Check sheet for the drawn part. Datum: minimum x, y, z corner. Units: mm. A direction names the side the tool comes from. Coordinates: 2 decimals unless noted, no trailing zeros. Loops run counter-clockwise (first coordinate to the right, second up) from the corner with the lowest first, then second, coordinate; pieces in that order, holes last. Notation, with made-up numbers: (60, 7.25) - (89, 7.25) arc R34 ccw to (89, 43.25) - close; hole circle Ø8 at (-4.5, 22.5). An arc over 180 degrees is marked (long way). Answer as CSV lines item,"result". Start each with the question number.
1. Cross-section at B-B (x = 9). Enter the section's corners in (y, z).
2. Cross-section at D-D (z = 4.25). Enter the section's corners in (x, y), plus the area to 3 significant figures.
3. Cross-section at A-A (y = 8). Enter the section's corners in (x, z), plus the area to 3 significant figures.
4. Cross-section at C-C (z = 6.25). Enter the section's corners in (x, y).
5. Gauge pin test, flat ends, axial feed: P1, Ø4, axis at x = 19, z = 5, coming from the -Y side; P2, Ø5, axis at x = 19.5, y = 17.5, coming from the +Z side. Record the tip position at first contact, or that the pin passes through.
6. Material ranges on line 1 (Y direction, x = 5, z = 0.4); line 2 (Y direction, x = 26.5, z = 4.5); line 3 (Z direction, x = 25, y = 24.5), recorded low to high. Write a range as [from, to].
7. Set-up check for the marked faces 1 and 2: record each of +Z, -Z, +X, -X, +Y, -Y from which the full face is reachable in a straight line by a thin tool's end or side.
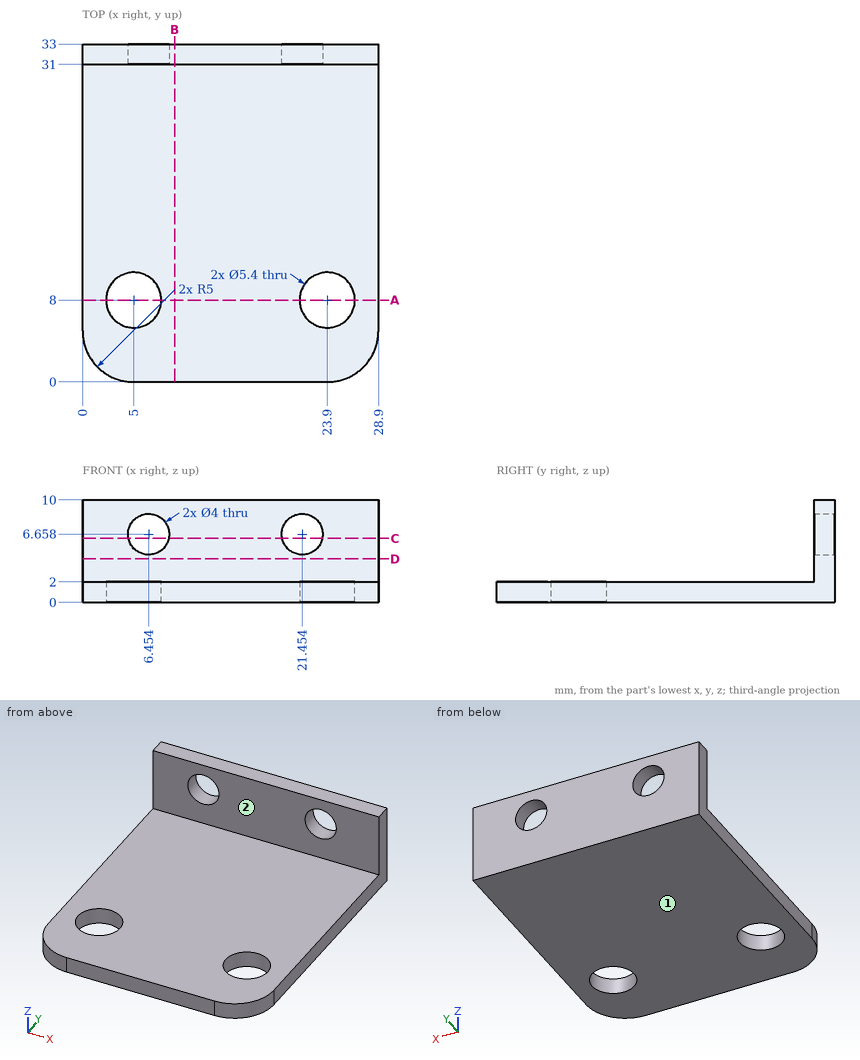
Values follow:
1,outline,"(0, 0) - (33, 0) - (33, 10) - (31, 10) - (31, 2) - (0, 2) - close"
2,outline,"(0, 31) - (28.9, 31) - (28.9, 33) - (0, 33) - close"
2,area,"57.8 mm²"
3,outline,"(0, 0) - (2.3, 0) - (2.3, 2) - (0, 2) - close; (7.7, 0) - (21.2, 0) - (21.2, 2) - (7.7, 2) - close; (26.6, 0) - (28.9, 0) - (28.9, 2) - (26.6, 2) - close"
3,area,"36.2 mm²"
4,outline,"(0, 31) - (4.5, 31) - (4.5, 33) - (0, 33) - close; (8.41, 31) - (19.5, 31) - (19.5, 33) - (8.41, 33) - close; (23.41, 31) - (28.9, 31) - (28.9, 33) - (23.41, 33) - close"
5,P1,"stops at y = 31"
5,P2,"stops at z = 2"
6,line 1,"y = [0, 5.3], [10.7, 33]"
6,line 2,"y = [31, 33]"
6,line 3,"z = [0, 2]"
7,face 1,"-Z, +X, -X, +Y, -Y"
7,face 2,"+Z, +X, -X, -Y"
